Design review of the part built by this model. Coordinates are the model's own, in mm. Coordinates: 2 decimals unless noted, no trailing zeros. Order: outer loops, then holes, each group sorted by start corner. A loop starts at its lowest first (then second) coordinate and runs counter-clockwise, first axis right, second up. Notation, with made-up numbers: (-27, -4.5) -> (25, -4.5) arc R15 cw to (25, 2.5) -> close; hole circle Ø10 at (86.5, -24.5). An arc over 180 degrees is marked (long way). Write item = value, one per line.
```python
from build123d import *

# Parameters (mm, degrees)
SKETCH1_R           = 3.3655
BOSS_EXTRUDE1_DEPTH = 9.525
SKETCH2_R           = 0.877000024
CUT_EXTRUDE1_DEPTH  = 10.525


with BuildPart() as part:
    # Sketch1 → Boss-Extrude1 (new body)
    with BuildSketch(Plane.XY):
        with BuildLine():
            Line((-6.35, 0), (-6.35, 82.55))
            ThreePointArc((-6.35, 82.55), (0, 88.9), (6.35, 82.55))
            Line((6.35, 82.55), (6.35, 0))
            ThreePointArc((6.35, 0), (0, -6.35), (-6.35, 0))
        make_face()
        with Locations((0, 82.55)):
            Circle(SKETCH1_R, mode=Mode.SUBTRACT)
        Circle(SKETCH1_R, mode=Mode.SUBTRACT)
    extrude(amount=BOSS_EXTRUDE1_DEPTH)

    # Sketch2 → Cut-Extrude1 (cut, through all)
    with BuildSketch(Plane.XY.offset(9.525)):
        with Locations((0, 6.99999997)):
            Circle(SKETCH2_R)
        with Locations((0, 16.000000004)):
            Circle(SKETCH2_R)
    extrude(amount=-CUT_EXTRUDE1_DEPTH, mode=Mode.SUBTRACT)


solid = part.part
```
(1) We need section D-D (x = -4.5). Write out the cut boundary in (y, z) (3 decimals).
Report:
outline = (-4.48, 0) -> (87.03, 0) -> (87.03, 9.525) -> (-4.48, 9.525) -> close
(2) Insertion check: pin 1 (2 mm diameter, centred on x = 1.5, z = 8.5, fed in from +Y); pin 2 (2 mm diameter, centred on x = -2.5, z = 8.5, fed in from +Y). Each pin has a flat end and moves straight along its axis. Give the tip position at first contact, or say it passes through.
Report:
pin_1 = 88.88
pin_2 = 88.72
(3) We need section B-B (x = 0). Give the number of separate pieces and of enclosed holes in the cut face, and give its area (3 significant figures).
Report:
separate_pieces = 5
enclosed_holes = 0
area = 746 mm²
(4) The part is to be moulded in two halves that separate along X. For faces 1 (the cylindrical face through (-0.1, 88.9, 4.7)), 2 (the flat face through (-6.35, 41, 5)), 3 (the flat face through (6.35, 42, 5)), 4 (the cylindrical face through (-0.438, 85.887, 4.696)), say which applies: released by +X, released by -X, zero draft, split by the parting line, or undercut.
Report:
face_1 = split by the parting line
face_2 = released by -X
face_3 = released by +X
face_4 = undercut
(5) We need section A-A (z = 8.25). Write out the cut boundary in (x, y), and give its area (3 significant figures).
Report:
outline = (-6.35, 0) arc R6.35 ccw to (6.35, 0) -> (6.35, 82.55) arc R6.35 ccw to (-6.35, 82.55) -> close; hole circle Ø6.73 at (0, 0); hole circle Ø6.73 at (0, 82.55); hole circle Ø1.75 at (0, 7); hole circle Ø1.75 at (0, 16)
area = 1,100 mm²
(6) We need section C-C (y = 16). Write out the cut boundary in (x, z) (3 decimals).
Report:
outline = (-6.35, 0) -> (-0.877, 0) -> (-0.877, 9.525) -> (-6.35, 9.525) -> close; (0.877, 0) -> (6.35, 0) -> (6.35, 9.525) -> (0.877, 9.525) -> close
(7) For L1, parallel to Y at x = 0, z = 7.75; L2, parallel to Y at x = 2.5, z = 1.75; L3, parallel to Y at x = -1, z = 4, list the stretches that pass through material, from the lowest coordinate up.
Report:
L1 = -6.35 to -3.37, 3.37 to 6.12, 7.88 to 15.12, 16.88 to 79.18, 85.92 to 88.9
L2 = -5.84 to -2.25, 2.25 to 80.3, 84.8 to 88.39
L3 = -6.27 to -3.21, 3.21 to 79.34, 85.76 to 88.82
